Read the model definition and answer for the solid it produces. Units are mm, in the model's axes. A direction names the side the tool comes from. Round coordinates to 2 decimals unless told otherwise and drop trailing zeros. Write each loop counter-clockwise with the first axis right and the second up, starting at its lowest first coordinate (ties: lowest second). Pieces come first, ordered by that corner, then holes. Notation, with made-up numbers: (38.25, 63) -> (61.25, 63) arc R23 ccw to (61.25, 95) -> close; hole circle Ø9 at (-3.75, 73). An arc over 180 degrees is marked (long way). Return JSON: item names as keys, results as strings. Group by question number.
(1) A cutting plane is placed at D-D on y = 6. Give the vertices of the cut face in (x, z).
(2) A cutting plane is placed at B-B on z = 4.8. Give the vertices of the cut face in (x, y), then the cut area to 3 significant figures.
(3) Straight lines are drawn through the part: line 1 (X direction, y = 2.75, z = 2.5); line 2 (X direction, y = -7.5, z = 2.2); line 3 (X direction, y = -7.5, z = 2.6). For each, find the intervals that lie inside material, in ascending order.
(4) A cutting plane is placed at A-A on y = -4.5. Give the vertices of the cut face in (x, z), then the cut area to 3 significant figures.
(5) For faces 1 (the flat face through (-8, 7.621, 5)), 2 (the flat face through (6.9, 0, 3)), 3 (the flat face through (0, 0, 4)), 4 (the cylindrical face through (0, -7, 2)), 5 (the flat face through (-8.95, 0, 5)), determine the directions among +Z, -Z, +X, -X, +Y, -Y from which every point of the face is accessible in a straight line to the end or side of a thin tool.
(6) A cutting plane is placed at C-C on x = 7.5. Give the vertices of the cut face in (y, z), then the cut area to 3 significant figures.
(7) The mould has two halves that part along Y. Classify faces 6 (the flat face through (-8, -7.379, 5)), 7 (the flat face through (-6.95, 0, 5)), 8 (the flat face through (8, 7.434, 3)), 9 (the flat face through (8, -7.766, 3)): released by +Y, released by -Y, zero draft, split by the parting line, or undercut.
(8) Given pin 1 (1.6 mm diameter, centred on x = 0, z = 3.5, fed in from -Y); pin 2 (1.5 mm diameter, centred on x = 6, y = -1.5, fed in from +Z); pin 3 (0.5 mm diameter, centred on y = -2.5, z = 4.5, fed in from -X), each flat-ended and moving along its own axis, determine where each tip first touches the part or whether it passes through.
```python
from build123d import *

# Parameters (mm, degrees)
SKETCH1_W               = 20
SKETCH1_H               = 20
BOSS_EXTRUDE1_DEPTH     = 4
SKETCH4_R               = 0.89
CUT_EXTRUDE1_DEPTH      = 0.25
CUT_EXTRUDE1_DEPTH_BACK = 8
SKETCH6_R               = 2
SKETCH7_W               = 2
SKETCH7_H               = 15
BOSS_EXTRUDE2_DEPTH     = 2
SKETCH8_W               = 2.1
SKETCH8_H               = 15.2
CUT_EXTRUDE2_DEPTH      = 2.5
FILLET1_R               = 0.25
FILLET2_R               = 0.25
FILLET3_R               = 0.25
FILLET5_R               = 0.5
FILLET6_R               = 0.5


with BuildPart() as part:
    # Sketch1 → Boss-Extrude1 (new body)
    with BuildSketch(Plane.XY):
        Rectangle(SKETCH1_W, SKETCH1_H)
    extrude(amount=BOSS_EXTRUDE1_DEPTH)

    # Sketch4 → Cut-Revolve1 (revolve, cut)
    with BuildSketch(Plane(origin=(0, 0, 0), x_dir=(1, 0, 0), z_dir=(0, 1, 0)), mode=Mode.PRIVATE) as cut_revolve1_sk:
        with Locations((3.125, -4)):
            Circle(SKETCH4_R)
    revolve(cut_revolve1_sk.sketch.rotate(Axis((0, 0, 0), (0, 0, 1)), 180), axis=Axis((0, 0, 0), (0, 0, 1)), mode=Mode.SUBTRACT)

    # Sketch6 → Cut-Extrude1 (cut, two sides: drawn at the far end of the back side and taken through both)
    with BuildSketch(Plane(origin=(0, -4, 0), x_dir=(1, 0, 0), z_dir=(0, 1, 0)).offset(-CUT_EXTRUDE1_DEPTH_BACK)):
        with Locations((0, -4)):
            Circle(SKETCH6_R)
    extrude(amount=CUT_EXTRUDE1_DEPTH + CUT_EXTRUDE1_DEPTH_BACK, mode=Mode.SUBTRACT)

    # Sketch7 → Boss-Extrude2 (add)
    with BuildSketch(Plane.XY.offset(4)):
        with Locations((-7.95, 0.121431972)):
            Rectangle(SKETCH7_W, SKETCH7_H)
    extrude(amount=BOSS_EXTRUDE2_DEPTH)

    # Sketch8 → Cut-Extrude2 (cut)
    with BuildSketch(Plane.XY.offset(4)):
        with Locations((7.95, -0.165781366)):
            Rectangle(SKETCH8_W, SKETCH8_H)
    extrude(amount=-CUT_EXTRUDE2_DEPTH, mode=Mode.SUBTRACT)

    # Fillet1
    fillet1_edges = [part.edges().sort_by_distance(p)[0] for p in [
        (-8.95, 0.121431972, 6),
        (-7.95, -7.378568028, 6),
        (-6.95, 0.121431972, 6),
        (-7.95, 7.621431972, 6),
    ]]
    fillet(fillet1_edges, radius=FILLET1_R)

    # Fillet2
    # the kernel refuses this fillet: 0.25 mm, written as the material it takes off along each edge
    with BuildSketch(Plane(origin=(-7.2, -7.128568028, 5.75), x_dir=(0, -1, 0), z_dir=(1, 0, 0))) as fillet2_piece_1_section:
        Polygon((0, 0), (FILLET2_R, 0), (FILLET2_R, -FILLET2_R), (0, -FILLET2_R), align=None)
    fillet2_piece_1 = extrude(amount=FILLET2_R, mode=Mode.PRIVATE)
    fillet2_piece_1 = fillet2_piece_1 - Plane(origin=(-7.2, -7.128568028, 5.75), x_dir=(0, 0.7071067811865475, -0.7071067811865475), z_dir=(1, 0, 0)) * Sphere(FILLET2_R, mode=Mode.PRIVATE)
    add(fillet2_piece_1, mode=Mode.SUBTRACT)
    with BuildSketch(Plane(origin=(-8.7, -7.128568028, 5.75), x_dir=(-1, 0, 0), z_dir=(0, -1, 0))) as fillet2_piece_2_section:
        Polygon((0, 0), (FILLET2_R, 0), (FILLET2_R, -FILLET2_R), (0, -FILLET2_R), align=None)
    fillet2_piece_2 = extrude(amount=FILLET2_R, mode=Mode.PRIVATE)
    fillet2_piece_2 = fillet2_piece_2 - Plane(origin=(-8.7, -7.128568028, 5.75), x_dir=(0.7071067811865475, 0, -0.7071067811865475), z_dir=(0, -1, 0)) * Sphere(FILLET2_R, mode=Mode.PRIVATE)
    add(fillet2_piece_2, mode=Mode.SUBTRACT)
    with BuildSketch(Plane(origin=(-7.2, 7.371431972, 5.75), x_dir=(0, 1, 0), z_dir=(1, 0, 0))) as fillet2_piece_3_section:
        Polygon((0, 0), (FILLET2_R, 0), (FILLET2_R, FILLET2_R), (0, FILLET2_R), align=None)
    fillet2_piece_3 = extrude(amount=FILLET2_R, mode=Mode.PRIVATE)
    fillet2_piece_3 = fillet2_piece_3 - Plane(origin=(-7.2, 7.371431972, 5.75), x_dir=(0, -0.7071067811865475, -0.7071067811865475), z_dir=(1, 0, 0)) * Sphere(FILLET2_R, mode=Mode.PRIVATE)
    add(fillet2_piece_3, mode=Mode.SUBTRACT)
    with BuildSketch(Plane(origin=(-8.7, 7.371431972, 5.75), x_dir=(-1, 0, 0), z_dir=(0, 1, 0))) as fillet2_piece_4_section:
        Polygon((0, 0), (FILLET2_R, 0), (FILLET2_R, FILLET2_R), (0, FILLET2_R), align=None)
    fillet2_piece_4 = extrude(amount=FILLET2_R, mode=Mode.PRIVATE)
    fillet2_piece_4 = fillet2_piece_4 - Plane(origin=(-8.7, 7.371431972, 5.75), x_dir=(0.7071067811865475, 0, -0.7071067811865475), z_dir=(0, 1, 0)) * Sphere(FILLET2_R, mode=Mode.PRIVATE)
    add(fillet2_piece_4, mode=Mode.SUBTRACT)
    with BuildSketch(Plane(origin=(-8.95, 7.621431972, 4), x_dir=(1, 0, 0), z_dir=(0, 0, 1)), Plane(origin=(-6.95, 7.621431972, 4), x_dir=(0, -1, 0), z_dir=(0, 0, 1))) as fillet2_piece_5:
        with BuildLine():
            CenterArc((FILLET2_R, -FILLET2_R), FILLET2_R, 90, 90)
            Line((0, -FILLET2_R), (0, 0))
            Line((0, 0), (FILLET2_R, 0))
        make_face()
    extrude(amount=1.75, mode=Mode.SUBTRACT)
    with BuildSketch(Plane(origin=(-6.95, -7.378568028, 4), x_dir=(0, 1, 0), z_dir=(0, 0, 1)), Plane(origin=(-8.95, -7.378568028, 4), x_dir=(1, 0, 0), z_dir=(0, 0, 1))) as fillet2_piece_6:
        with BuildLine():
            CenterArc((FILLET2_R, FILLET2_R), FILLET2_R, 180, 90)
            Line((0, FILLET2_R), (0, 0))
            Line((0, 0), (FILLET2_R, 0))
        make_face()
    extrude(amount=1.75, mode=Mode.SUBTRACT)

    # Fillet3
    fillet3_edges = [part.edges().sort_by_distance(p)[0] for p in [
        (6.9, -0.165781366, 4),
        (7.95, -7.765781366, 4),
        (9, -0.165781366, 4),
        (7.95, 7.434218634, 4),
    ]]
    fillet(fillet3_edges, radius=FILLET3_R)

    # Fillet5
    fillet5_edges = [part.edges().sort_by_distance(p)[0] for p in [
        (0, 10, 0),
        (10, 0, 0),
        (0, -10, 0),
        (-10, 0, 0),
    ]]
    fillet(fillet5_edges, radius=FILLET5_R)

    # Fillet6
    # the kernel refuses this fillet: 0.5 mm, written as the material it takes off along each edge
    with BuildSketch(Plane(origin=(-9.5, 9.5, 0.5), x_dir=(-1, 0, 0), z_dir=(0, 1, 0))) as fillet6_piece_1_section:
        Polygon((0, 0), (FILLET6_R, 0), (FILLET6_R, -FILLET6_R), (0, -FILLET6_R), align=None)
    fillet6_piece_1 = extrude(amount=FILLET6_R, mode=Mode.PRIVATE)
    fillet6_piece_1 = fillet6_piece_1 - Plane(origin=(-9.5, 9.5, 0.5), x_dir=(0.7071067811865475, 0, 0.7071067811865475), z_dir=(0, 1, 0)) * Sphere(FILLET6_R, mode=Mode.PRIVATE)
    add(fillet6_piece_1, mode=Mode.SUBTRACT)
    with BuildSketch(Plane(origin=(9.5, 9.5, 0.5), x_dir=(0, 1, 0), z_dir=(1, 0, 0))) as fillet6_piece_2_section:
        Polygon((0, 0), (FILLET6_R, 0), (FILLET6_R, -FILLET6_R), (0, -FILLET6_R), align=None)
    fillet6_piece_2 = extrude(amount=FILLET6_R, mode=Mode.PRIVATE)
    fillet6_piece_2 = fillet6_piece_2 - Plane(origin=(9.5, 9.5, 0.5), x_dir=(0, -0.7071067811865475, 0.7071067811865475), z_dir=(1, 0, 0)) * Sphere(FILLET6_R, mode=Mode.PRIVATE)
    add(fillet6_piece_2, mode=Mode.SUBTRACT)
    with BuildSketch(Plane(origin=(-9.5, -9.5, 0.5), x_dir=(-1, 0, 0), z_dir=(0, -1, 0))) as fillet6_piece_3_section:
        Polygon((0, 0), (FILLET6_R, 0), (FILLET6_R, FILLET6_R), (0, FILLET6_R), align=None)
    fillet6_piece_3 = extrude(amount=FILLET6_R, mode=Mode.PRIVATE)
    fillet6_piece_3 = fillet6_piece_3 - Plane(origin=(-9.5, -9.5, 0.5), x_dir=(0.7071067811865475, 0, 0.7071067811865475), z_dir=(0, -1, 0)) * Sphere(FILLET6_R, mode=Mode.PRIVATE)
    add(fillet6_piece_3, mode=Mode.SUBTRACT)
    with BuildSketch(Plane(origin=(9.5, -9.5, 0.5), x_dir=(0, -1, 0), z_dir=(1, 0, 0))) as fillet6_piece_4_section:
        Polygon((0, 0), (FILLET6_R, 0), (FILLET6_R, FILLET6_R), (0, FILLET6_R), align=None)
    fillet6_piece_4 = extrude(amount=FILLET6_R, mode=Mode.PRIVATE)
    fillet6_piece_4 = fillet6_piece_4 - Plane(origin=(9.5, -9.5, 0.5), x_dir=(0, 0.7071067811865475, 0.7071067811865475), z_dir=(1, 0, 0)) * Sphere(FILLET6_R, mode=Mode.PRIVATE)
    add(fillet6_piece_4, mode=Mode.SUBTRACT)
    with BuildSketch(Plane(origin=(-10, 10, 0.5), x_dir=(1, 0, 0), z_dir=(0, 0, 1)), Plane(origin=(10, 10, 0.5), x_dir=(0, -1, 0), z_dir=(0, 0, 1))) as fillet6_piece_5:
        with BuildLine():
            CenterArc((FILLET6_R, -FILLET6_R), FILLET6_R, 90, 90)
            Line((0, -FILLET6_R), (0, 0))
            Line((0, 0), (FILLET6_R, 0))
        make_face()
    extrude(amount=4.75, mode=Mode.SUBTRACT)
    with BuildSketch(Plane(origin=(10, -10, 0.5), x_dir=(0, 1, 0), z_dir=(0, 0, 1)), Plane(origin=(-10, -10, 0.5), x_dir=(1, 0, 0), z_dir=(0, 0, 1))) as fillet6_piece_6:
        with BuildLine():
            CenterArc((FILLET6_R, FILLET6_R), FILLET6_R, 180, 90)
            Line((0, FILLET6_R), (0, 0))
            Line((0, 0), (FILLET6_R, 0))
        make_face()
    extrude(amount=4.75, mode=Mode.SUBTRACT)


solid = part.part
```
Checks:
{
 "1": {"outline": "(-10, 0.5) arc R0.5 ccw to (-9.5, 0) -> (9.5, 0) arc R0.5 ccw to (10, 0.5) -> (10, 4) -> (9.25, 4) arc R0.25 ccw to (9, 3.75) -> (9, 1.5) -> (6.9, 1.5) -> (6.9, 3.75) arc R0.25 ccw to (6.65, 4) -> (-6.95, 4) -> (-6.95, 5.75) arc R0.25 ccw to (-7.2, 6) -> (-8.7, 6) arc R0.25 ccw to (-8.95, 5.75) -> (-8.95, 4) -> (-10, 4) -> close"},
 "2": {"outline": "(-8.95, -7.13) arc R0.25 ccw to (-8.7, -7.38) -> (-7.2, -7.38) arc R0.25 ccw to (-6.95, -7.13) -> (-6.95, 7.37) arc R0.25 ccw to (-7.2, 7.62) -> (-8.7, 7.62) arc R0.25 ccw to (-8.95, 7.37) -> close", "area": "29.9 mm^2"},
 "3": {"line 1": "x = -10 to 6.9, 9 to 10", "line 2": "x = -10 to -0.87, 0.87 to 6.9, 9 to 10", "line 3": "x = -10 to -1.43, 1.43 to 6.9, 9 to 10"},
 "4": {"outline": "(-10, 0.5) arc R0.5 ccw to (-9.5, 0) -> (9.5, 0) arc R0.5 ccw to (10, 0.5) -> (10, 4) -> (9.25, 4) arc R0.25 ccw to (9, 3.75) -> (9, 1.5) -> (6.9, 1.5) -> (6.9, 3.75) arc R0.25 ccw to (6.65, 4) -> (2, 4) arc R2 cw to (-2, 4) -> (-6.95, 4) -> (-6.95, 5.75) arc R0.25 ccw to (-7.2, 6) -> (-8.7, 6) arc R0.25 ccw to (-8.95, 5.75) -> (-8.95, 4) -> (-10, 4) -> close", "area": "72.3 mm^2"},
 "5": {"face 1": "+Z, +X, -X, +Y", "face 2": "+Z", "face 3": "+Z, +X, +Y, -Y", "face 4": "+Z, -Y", "face 5": "+Z, -X, +Y, -Y"},
 "6": {"outline": "(-10, 0.5) arc R0.5 ccw to (-9.5, 0) -> (9.5, 0) arc R0.5 ccw to (10, 0.5) -> (10, 4) -> (7.68, 4) arc R0.25 ccw to (7.43, 3.75) -> (7.43, 1.5) -> (-7.77, 1.5) -> (-7.77, 3.75) arc R0.25 ccw to (-8.02, 4) -> (-10, 4) -> close", "area": "41.9 mm^2"},
 "7": {"face 6": "released by -Y", "face 7": "zero draft", "face 8": "undercut", "face 9": "undercut"},
 "8": {"pin 1": "stops at y = -3.75", "pin 2": "stops at z = 4", "pin 3": "stops at x = -8.95"}
}
